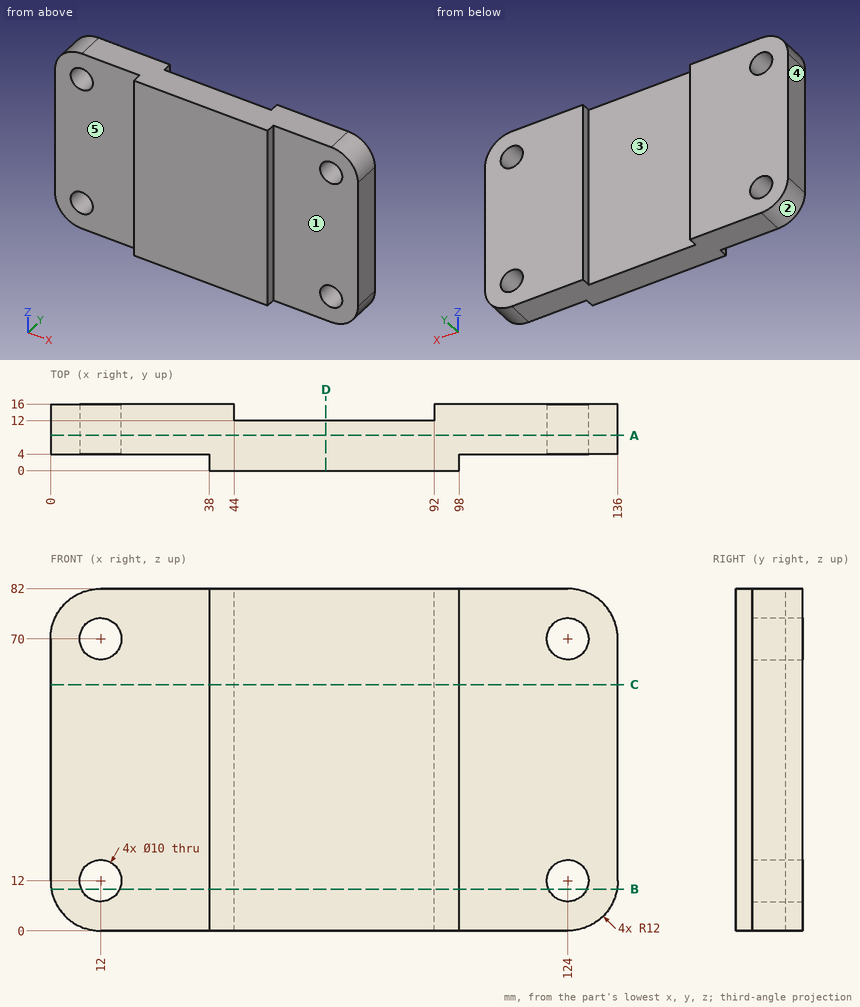
Verification items for this drawing (mm, ordinates from the low corner). A direction names the side the tool comes from. Give positions to 0.01 mm unless a question says otherwise; leave off trailing zeros. Loops run counter-clockwise (first coordinate to the right, second up) from the corner with the lowest first, then second, coordinate; pieces in that order, holes last. Notation, with made-up numbers: (10, 23) - (56, 23) arc R18 cw to (56, 32) - close; hole circle Ø7 at (14.5, 22.25). An arc over 180 degrees is marked (long way). Write item = value, one per line. Start each with the question number.
Q1. Cross-section at C-C, the plane z = 59. Enter the section's corners in (x, y).
Q2. Mould release check, pull along X, two halves, no side actions. Record for the marked faces 1, 2 and 3: released by +X, released by -X, zero draft, split by the parting line, or undercut.
Q3. Cross-section at D-D, the plane x = 66. Enter the section's corners in (y, z), and give its area (3 significant figures).
Q4. Depth check by flat-ended pin: P1, Ø4, axis at y = 3, z = 14, coming from the -X side; P2, Ø1, axis at x = 78.5, z = 41, coming from the +Y side; P3, Ø3, axis at y = 2, z = 27, coming from the -X side; P4, Ø3, axis at y = 14, z = 9, coming from the +X side. Enter the tip coordinate at first touch or a pass-through.
Q5. Cross-section at A-A, the plane y = 8.5. Enter the section's corners in (x, z).
Q6. Cross-section at B-B, the plane z = 10. Enter the section's corners in (x, y), and give its area (3 significant figures).
Q7. Thickness scan on line 1 (Z direction, x = 124, y = 8.5); line 2 (X direction, y = 12.25, z = 8); line 3 (Y direction, x = 53.5, z = 37.5). Record the ranges inside material, lowest first.
Q8. Tool access check on the marked faces 4 and 5. Record the directions out of +Z, -Z, +X, -X, +Y, -Y that give a thin tool (end or side, any length) a straight path to the whole face; none if there is none.
Answer key:
q1.outline = (0, 4) - (38, 4) - (38, 0) - (98, 0) - (98, 4) - (136, 4) - (136, 16) - (92, 16) - (92, 12) - (44, 12) - (44, 16) - (0, 16) - close
q2.face_1 = zero draft
q2.face_2 = released by -X
q2.face_3 = undercut
q3.outline = (0, 0) - (12, 0) - (12, 82) - (0, 82) - close
q3.area = 984 mm^2
q4.P1 = 0
q4.P2 = 12
q4.P3 = 38
q4.P4 = 135.91
q5.outline = (0, 12) arc R12 ccw to (12, 0) - (124, 0) arc R12 ccw to (136, 12) - (136, 70) arc R12 ccw to (124, 82) - (12, 82) arc R12 ccw to (0, 70) - close; hole circle Ø10 at (12, 12); hole circle Ø10 at (12, 70); hole circle Ø10 at (124, 12); hole circle Ø10 at (124, 70)
q6.outline = (0.17, 4) - (7.42, 4) - (7.42, 16) - (0.17, 16) - close; (16.58, 4) - (38, 4) - (38, 0) - (98, 0) - (98, 4) - (119.42, 4) - (119.42, 16) - (92, 16) - (92, 12) - (44, 12) - (44, 16) - (16.58, 16) - close; (128.58, 4) - (135.83, 4) - (135.83, 16) - (128.58, 16) - close
q6.area = 1,460 mm^2
q7.line_1 = 0 to 7, 17 to 65, 75 to 82
q7.line_2 = 0.69 to 9, 15 to 44, 92 to 121, 127 to 135.31
q7.line_3 = 0 to 12
q8.face_4 = +Z, -Z, -X, +Y, -Y
q8.face_5 = +Z, -Z, -X, -Y
